Check sheet for the modelled part. Datum: model origin and axes. Units: mm. A direction names the side the tool comes from. Give positions to 0.01 mm unless a question says otherwise; leave off trailing zeros. Write each loop counter-clockwise with the first axis right and the second up, starting at its lowest first coordinate (ties: lowest second). Pieces come first, ordered by that corner, then holes. Notation, with made-up numbers: (-6, -17) -> (46, -17) arc R26 cw to (46, 11) -> close; hole circle Ø7 at (20, -29). An arc over 180 degrees is marked (long way). Answer as a JSON object with one key per item and string values.
from build123d import *

# Parameters (mm, degrees)
F0_W      = 56.1024434865
F0_H      = 50.5313724279
F1_DEPTH  = 75.692
F2_DEPTH  = 140.716
F3_DEPTH  = 105.664
F4_R      = 78.7850873133
F5_DEPTH  = 190.246
F6_R      = 25.2857639188
F7_DEPTH  = 125.476
F8_R      = 34.6183044946
F9_DEPTH  = 83.566
F11_DEPTH = 167.386


with BuildPart() as f1:
    # F0 (on Front) → F1 (new body)
    with BuildSketch(Plane.XZ):
        with Locations((28.0512217432, 25.265686214)):
            Rectangle(F0_W, F0_H)
    extrude(amount=F1_DEPTH)

    # F2 (add): a face of the model
    f2_faces = [f1.faces().sort_by_distance(p)[0] for p in [
        (56.1024434865, -37.846, 25.265686214),
    ]]
    extrude(f2_faces, amount=F2_DEPTH)

    # F3 (add): a face of the model
    f3_faces = [f1.faces().sort_by_distance(p)[0] for p in [
        (98.4092217432, -75.692, 25.265686214),
    ]]
    extrude(f3_faces, amount=F3_DEPTH)

    # F4 (on face) → F5 (join)
    with BuildSketch(Plane.XY.offset(50.5313724279)):
        with Locations((95.3895151615, -95.1104015112)):
            Circle(F4_R)
    extrude(amount=F5_DEPTH)

    # F6 (on face) → F7 (cut)
    with BuildSketch(Plane.XY.offset(240.7773724279)):
        with Locations((95.3895151615, -95.1104015112)):
            Circle(F6_R)
    extrude(amount=F7_DEPTH, mode=Mode.SUBTRACT)

    # F8 (on face) → F9 (cut)
    with BuildSketch(Plane.XY.offset(240.7773724279)):
        with Locations((95.3895151615, -95.1104015112)):
            Circle(F8_R)
    extrude(amount=-F9_DEPTH, mode=Mode.SUBTRACT)

    # F10 (on face) → F11 (cut)
    with BuildSketch(Plane.XY.offset(240.7773724279)):
        Polygon((40.0986362787, -144.27217879), (125.0593225865, -162.8869768172), (169.0173434726, -87.8368514126), (111.2242081507, -22.8385250253), (31.5480653191, -57.7174755108), align=None)
    extrude(amount=-F11_DEPTH, mode=Mode.SUBTRACT)


solid = f1.part
1. Go/stop test with flat-tipped pins: P1, Ø6, axis at y = -87.5, z = 140.5, coming from the +X side; P2, Ø6, axis at x = 90, y = -148.5, coming from the +Z side; P3, Ø3, axis at x = 58, z = 62.5, coming from the +Y side. Record where each tip stops, or that it passes through.
Determined:
{"P1": "x = 174.04", "P2": "z = 73.39", "P3": "y = -24.97"}
2. Sectioned sample at D-D, the plane x = 183. Enter the section's corners in (y, z).
Determined:
{"outline": "(-181.36, 0) -> (0, 0) -> (0, 50.53) -> (-181.36, 50.53) -> close"}
3. Sectioned sample at B-B, the plane x = 130. Enter the section's corners in (y, z), plus the area to 3 significant figures.
Determined:
{"outline": "(-181.36, 0) -> (0, 0) -> (0, 50.53) -> (-24.33, 50.53) -> (-24.33, 240.78) -> (-43.96, 240.78) -> (-43.96, 73.39) -> (-154.45, 73.39) -> (-154.45, 240.78) -> (-165.89, 240.78) -> (-165.89, 50.53) -> (-181.36, 50.53) -> close", "area": "17,600 mm^2"}
4. Access from +Z, -Z, +X, -X, +Y, -Y to the whole of each face (thin tool, end or side, straight path). Record for faces 5 (the face through (71.944, -40.034, 158.256)), 6 (the face through (97, 0, 25)).
Determined:
{"face 5": "+Z", "face 6": "+Z, -Z, +X, -X, +Y"}
5. Mould release check, pull along X, two halves, no side actions. Record for faces 1 (the face through (100, -89, 0)), 2 (the face through (140.525, -55.793, 158.256)), 3 (the face through (99, -92, 73.391)), 4 (the face through (0, -89, 25)): released by +X, released by -X, zero draft, split by the parting line, or undercut.
Determined:
{"face 1": "zero draft", "face 2": "undercut", "face 3": "undercut", "face 4": "released by -X"}
6. Scan lines: L1, parallel to Z at x = 146, y = -15; L2, parallel to X at y = -33, z = 205; L3, parallel to Y at x = 76.5, z = 220. Record each from-to range of solid material in increasing order. Write a range as [from, to].
Determined:
{"L1": "[0, 50.53]", "L2": "[46.92, 88.01], [120.26, 143.86]", "L3": "[-171.6, -152.25], [-38.04, -18.62]"}
7. Sectioned sample at A-A, the plane z = 216. Enter the section's corners in (x, y).
Determined:
{"outline": "circle Ø157.57 at (95.39, -95.11); hole (31.55, -57.72) -> (40.1, -144.27) -> (125.06, -162.89) -> (169.02, -87.84) -> (111.22, -22.84) -> close"}
8. Sectioned sample at C-C, the plane y = -38.5. Enter the section's corners in (x, z), plus the area to 3 significant figures.
Determined:
{"outline": "(0, 0) -> (196.82, 0) -> (196.82, 50.53) -> (150.18, 50.53) -> (150.18, 240.78) -> (125.15, 240.78) -> (125.15, 73.39) -> (75.45, 73.39) -> (75.45, 240.78) -> (40.6, 240.78) -> (40.6, 50.53) -> (0, 50.53) -> close", "area": "22,500 mm^2"}
